Autodesk Inventor part; units mm, degrees
ref_plane "Work Plane3" through (24.6779, 24, 0) normal (0, 1, 0) x (1, 0, 0)
ref_plane "Work Plane4" through (5, 25.5147, -6) normal (1, 0, 0) x (0, 0, -1)
ref_plane "Work Plane2" through (0, 0, 0) normal (0.7071, -0.7071, 0) x (0, 0, -1)
sketch "Sketch1" plane through (0, 0, 0) normal (0, 0, 1) x (1, 0, 0)
  arc A0 (23.1619, 2.0217) -> (23.1619, -2.0217) centre (0, 0) ccw
  arc A1 (25.5104, 5.0217) -> (25.5104, -5.0217) centre (0, 0) ccw
  line L0 (23.1619, 2.0217) -> (35.5104, 2.0217)
  line L1 (25.5104, 5.0217) -> (35.5104, 5.0217)
  line L2 (35.5104, 5.0217) -> (35.5104, 2.0217)
  line L3 (0, 0) -> (18.0567, 0)
  line L4 (23.1619, -2.0217) -> (35.5104, -2.0217)
  line L5 (25.5104, -5.0217) -> (35.5104, -5.0217)
  line L6 (35.5104, -5.0217) -> (35.5104, -2.0217)
  dimension "d0" = 46.5
  dimension "d1" = 52
  dimension "d33" = 3
  dimension "d34" = 10
extrude "Extrusion1" add sketch "Sketch1" against normal blind 10
sketch "Sketch2" plane through (24.6779, 5.0217, 0) normal (0, 1, 0) x (1, 0, 0)
  line L0 (10.8325, 0) -> (0.8325, 0)
  line L1 (10.8325, 0) -> (10.8325, 10)
  line L2 (0.8325, 10) -> (10.8325, 10)
  line L3 (0.8325, 0) -> (0.8325, 10)
  circle A0 centre (5.8325, 5) radius 2
  point P0 (-24.6779, 0)
  dimension "d35" = 4
extrude "Extrusion2" cut sketch "Sketch2" against normal blind 11 contours A0
ref_plane "Work Plane3" through (24.6779, 24, 0) normal (0, 1, 0) x (1, 0, 0)
sketch "Sketch3" plane through (24.6779, 24, 0) normal (0, 1, 0) x (1, 0, 0)
  line L0 (-24.6779, 0) -> (-24.6779, 10)
  line L1 (-19.6779, 7.5) -> (-29.6779, 7.5)
  line L2 (-29.6779, 2.5) -> (-19.6779, 2.5)
  line L3 (-19.6779, 2.5) -> (-19.6779, 7.5)
  line L4 (-29.6779, 2.5) -> (-29.6779, 7.5)
  point P0 (-24.6779, 5)
extrude "Extrusion3" add sketch "Sketch3" along normal blind 22.5
ref_plane "Work Plane4" through (5, 25.5147, -6) normal (1, 0, 0) x (0, 0, -1)
sketch "Sketch4" plane through (5, 25.5147, -6) normal (1, 0, 0) x (0, 0, -1)
  line L0 (-3.5, 20.9853) -> (1.5, 20.9853)
  line L1 (-3.5, 20.9853) -> (11.5, 20.9853)
  line L2 (11.5, 20.9853) -> (11.5, 23.9853)
  line L3 (11.5, 23.9853) -> (-3.5, 23.9853)
  line L4 (-3.5, 23.9853) -> (-3.5, 20.9853)
  point P0 (-6, -24.4949)
  dimension "d36" = 15
  dimension "d37" = 3
extrude "Extrusion4" add sketch "Sketch4" against normal blind 10
ref_plane "Work Plane2" through (0, 0, 0) normal (0.7071, -0.7071, 0) x (0, 0, -1)
sketch "Sketch5" plane through (5, 49.5, -2.5) normal (0, 1, 0) x (1, 0, 0)
  circle A0 centre (-5, 10) radius 2
  dimension "d29" = 4
extrude "Extrusion5" cut sketch "Sketch5" against normal blind 4
fillet "Fillet2" radius 3 3 edges at (0, 49.5, -2.5) (5, 48, -17.5) (-5, 48, -17.5)
mirror "Mirror3" about plane through (0, 0, 0) normal (0, 1, 0) of "Extrusion4", "Fillet2", "Extrusion3", "Extrusion5"
properties part number "SupportBracket_v2_BilgePumpMotor" material "ABS Plastic"
Read the model definition and answer for the solid it produces. Units are mm, in the model's axes. A direction names the side the tool comes from. Give positions to 0.01 mm unless a question says otherwise; leave off trailing zeros. Write each loop counter-clockwise with the first axis right and the second up, starting at its lowest first coordinate (ties: lowest second). Pieces come first, ordered by that corner, then holes. Notation, with made-up numbers: (-6.75, 48) -> (26.25, 48) arc R28 cw to (26.25, 82) -> close; hole circle Ø10 at (50.5, 21). An arc over 180 degrees is marked (long way). Answer as a JSON object with one key per item and string values. Group by question number.
1) Find section B-B (z = -12.5). Write down the section's boundary in (x, y).
2) The mould has two halves that part along Z. Classify faces 4 (the cylindrical face through (-0.07, 48.6, -3.36)), 5 (the flat face through (0, -46.5, -10)), 6 (the cylindrical face through (28.512, 3.543, -5.088)), 7 (the cylindrical face through (-0.26, -48.021, -10.517)): +Z half, -Z half, draft (parallel to the pull), parting line (faces both ways), or undercut.
3) Find section D-D (y = 38). Write down the section's boundary in (x, z), and give its area (3 significant figures).
4) Consider L1, parallel to X at y = 47.45, z = -12.5; L2, parallel to X at y = -3.45, z = -5; L3, parallel to X at y = 4.4, z = -5. Determine where each line is inside the solid, lowest interval first. Write a range as from..to.
5) A tool of negligible diameter and unlimited length cuts with its end or side. For faces 1 (the flat face through (28, 5.022, -5)), 2 (the flat face through (23, 6, -10)), 3 (the flat face through (-5, 38, -6)), from which of +Z, -Z, +X, -X, +Y, -Y can it reach the whole face along a straight path? Write none if from no direction.
6) Find section A-A (x = 0). Count the separate pieces of the cut face and the enclosed holes in it, and give its area (3 significant figures).
7) Find section C-C (x = 16.5). Write down the section's boundary in (y, z).
8) Each of these flat-tipped pins is pushed along its axis until it touches: P1, Ø5, axis at x = 29.5, z = -7, coming from the +Y side; P2, Ø1.5, axis at y = -30, z = -7, coming from the +X side; P3, Ø3, axis at x = -16, z = -10, coming from the +Y side; P4, Ø2, axis at y = 26, z = -11.5, coming from the +X side. Where does it stop, or does it pass through?
Values follow:
{
 "1": {"outline": "(-5, -49.5) -> (-2, -49.5) -> (-2, -46.5) -> (-5, -46.5) -> close; (-5, 46.5) -> (-2, 46.5) -> (-2, 49.5) -> (-5, 49.5) -> close; (2, -49.5) -> (5, -49.5) -> (5, -46.5) -> (2, -46.5) -> close; (2, 46.5) -> (5, 46.5) -> (5, 49.5) -> (2, 49.5) -> close"},
 "2": {"face 4": "+Z half", "face 5": "draft", "face 6": "undercut", "face 7": "undercut"},
 "3": {"outline": "(-5, -7.5) -> (5, -7.5) -> (5, -2.5) -> (-5, -2.5) -> close", "area": "50.0 mm2"},
 "4": {"L1": "x = -5..-2, 2..5", "L2": "x = -25.77..-22.99, 22.99..28.51, 32.51..35.51", "L3": "x = -25.62..-22.83, 22.83..28.51, 32.51..35.51"},
 "5": {"face 1": "+Z, -Z, +X, +Y", "face 2": "-Z, +X, -X", "face 3": "+Z, -Z, -X, +Y"},
 "6": {"separate pieces": "4", "enclosed holes": "0", "area": "322 mm2"},
 "7": {"outline": "(-20.09, -10) -> (-16.38, -10) -> (-16.38, 0) -> (-20.09, 0) -> close; (16.38, -10) -> (20.09, -10) -> (20.09, 0) -> (16.38, 0) -> close"},
 "8": {"P1": "stops at y = 5.02", "P2": "stops at x = 5", "P3": "stops at y = 21.58", "P4": "passes through"}
}
